The model under review builds one solid part; all positions refer to its coordinate system, in mm. Face numbers are marked on the shaded views. A direction names the side the tool comes from. Give positions to 0.01 mm unless a question says otherwise; leave off trailing zeros. Loops run counter-clockwise (first coordinate to the right, second up) from the corner with the lowest first, then second, coordinate; pieces in that order, holes last. Notation, with made-up numbers: M 83.5,-36.5 L 96.5,-36.5 A30 cw 96.5,-8.5 Z; hole C 68,-18.5 d5. An arc over 180 degrees is marked long. One line per item, written item: value. Start each with the question number.
Q1. To check wall thickness, follow line 1 along X through (y, z) = (-6, 22.5); line 2 along X through (y, z) = (-11, 19); line 3 along X through (y, z) = (-14, 16.25). State the ranges of each line that lie inside material, in increasing order. Write a range as from..to.
Q2. For the marked faces 1, 2 and 3, list the 3-axis set-ups (+Z, -Z, +X, -X, +Y, -Y) from which the entire face can be reached by the end or side of a thin tool; tool diameter is ignored.
Q3. We need section C-C on y = -5.5. Write out the cut boundary in (x, z), plus the area to 3 significant figures.
Q4. We need section B-B on x = 2. Write out the cut boundary in (y, z).
Q5. For pin 1 (15 mm diameter, centred on x = 33.5, y = -12, fed in from +Z); pin 2 (4 mm diameter, centred on y = 21, z = 23, fed in from +X); pin 3 (8 mm diameter, centred on x = 71, z = 14, fed in from +Y); pin 4 (8 mm diameter, centred on x = 98.5, y = -15, fed in from -Z), all flat-tipped, find the tip position at first contact; note any pin that passes through.
Q6. We need section A-A on z = 12.5. Write out the cut boundary in (x, y).
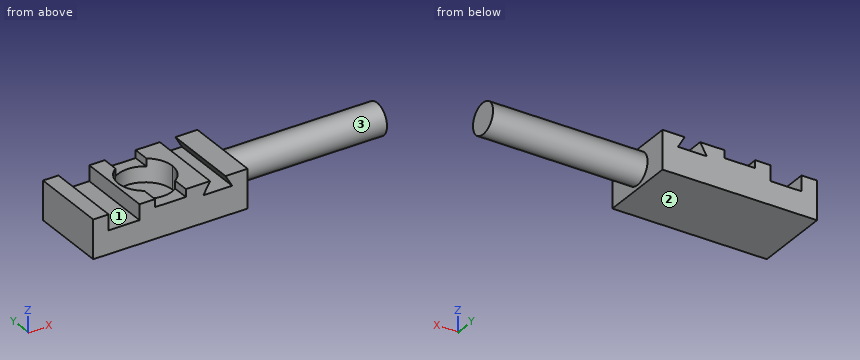
```python
from build123d import *

# Parameters (mm, degrees)
F0_W      = 100
F0_H      = 50
F1_DEPTH  = 25
F2_W      = 20
F2_H      = 50
F3_DEPTH  = 10
F4_DEPTH  = 5
F6_DEPTH  = 50
F7_R      = 10
F8_DEPTH  = 100
F10_DEPTH = 15


# Not quite as in the source:
# - a feature names something its author has since deleted; it is built from what else it names


with BuildPart() as f1:
    # F0 (on Top) → F1 (new body)
    with BuildSketch(Plane.XY):
        Rectangle(F0_W, F0_H)
    extrude(amount=F1_DEPTH)

    # F2 (on face) → F3 (cut)
    with BuildSketch(Plane.XY.offset(25)):
        with Locations((-30, 0)):
            Rectangle(F2_W, F2_H)
    extrude(amount=-F3_DEPTH, mode=Mode.SUBTRACT)

    # F2 (on face) → F4 (cut)
    with BuildSketch(Plane.XY.offset(25)):
        Rectangle(F2_W, F2_H)
    extrude(amount=-F4_DEPTH, mode=Mode.SUBTRACT)

    # F5 (on face) → F6 (cut, through all)
    with BuildSketch(Plane.XZ.offset(25)):
        Polygon((35.6698729811, 25), (25.6698729811, 25), (21.3397459622, 17.5), (40, 17.5), align=None)
    extrude(amount=-F6_DEPTH, mode=Mode.SUBTRACT)

    # F7 (on face) → F8 (join)
    with BuildSketch(Plane.YZ.offset(50)):
        with Locations((0, 12.5)):
            Circle(F7_R)
    extrude(amount=F8_DEPTH)

    # F9 (on face) → F10 (cut)
    with BuildSketch(Plane.XY.offset(25)):
        with BuildLine():
            ThreePointArc((-10, -14.3614066163), (8.100925873, -15.5120920575), (17.5, 0))
            ThreePointArc((17.5, 0), (8.100925873, 15.5120920575), (-10, 14.3614066163))
            Line((-10, 14.3614066163), (-10, -14.3614066163))
        make_face()
        with BuildLine():
            Line((-10, -14.3614066163), (-10, 14.3614066163))
            ThreePointArc((-10, 14.3614066163), (-17.5, 0), (-10, -14.3614066163))
        make_face()
    extrude(amount=-F10_DEPTH, mode=Mode.SUBTRACT)


solid = f1.part
```
Solved:
1. line 1: -50..-40, -20..-16.44, 16.44..24.23, 37.11..50
1. line 2: -50..-40, -20..-13.61, 13.61..22.21, 39.13..50
1. line 3: -50..-40, -20..-10.5, 10.5..50
2. face 1: +Z, +Y, -Y
2. face 2: -Z, +X, -X, +Y, -Y
2. face 3: +X
3. outline: M -50,0 L 50,0 L 50,4.15 L 150,4.15 L 150,20.85 L 50,20.85 L 50,25 L 35.67,25 L 40,17.5 L 21.34,17.5 L 25.67,25 L 16.61,25 L 16.61,10 L -16.61,10 L -16.61,25 L -20,25 L -20,15 L -40,15 L -40,25 L -50,25 Z
3. area: 3,360 mm2
4. outline: M -25,0 L 25,0 L 25,20 L 17.39,20 L 17.39,10 L -17.39,10 L -17.39,20 L -25,20 Z
5. pin 1: z = 25
5. pin 2: x = 50
5. pin 3: y = 10
5. pin 4: through
6. outline: M -50,-25 L 50,-25 L 50,-10 L 150,-10 L 150,10 L 50,10 L 50,25 L -50,25 Z; hole C 0,0 d35
